from build123d import *

# Parameters (mm, degrees)
SKETCH1_R               = 1.65
SKETCH1_W               = 45
SKETCH1_H               = 23.8
BOSS_EXTRUDE1_DEPTH     = 60
FILLET1_R               = 1.5
SKETCH2_W               = 2.5
SKETCH2_H               = 4.6
CUT_EXTRUDE1_DEPTH      = 10.5
FILLET2_R               = 1
CHAMFER1_SIZE           = 1
FILLET2_OF_MIRROR2_R    = 1
CHAMFER2_SIZE           = 1
CUT_EXTRUDE2_DEPTH      = 78.903850996
CUT_EXTRUDE2_DEPTH_BACK = 78.903850996


with BuildPart() as part:
    # Sketch1 → Boss-Extrude1 (new body)
    with BuildSketch(Plane.XY):
        Polygon((-25, -11.7), (-37.5, -11.7), (-37.5, -16.3), (37.5, -16.3), (37.5, -11.7), (25, -11.7), (25, 11.7), (37.5, 11.7), (37.5, 16.3), (-37.5, 16.3), (-37.5, 11.7), (-25, 11.7), align=None)
        with Locations((-31.25, -13.85)):
            Circle(SKETCH1_R, mode=Mode.SUBTRACT)
        with Locations((31.25, -13.85)):
            Circle(SKETCH1_R, mode=Mode.SUBTRACT)
        with Locations((0, -0.4)):
            Rectangle(SKETCH1_W, SKETCH1_H, mode=Mode.SUBTRACT)
        with Locations((-31.25, 13.85)):
            Circle(SKETCH1_R, mode=Mode.SUBTRACT)
        with Locations((31.25, 13.85)):
            Circle(SKETCH1_R, mode=Mode.SUBTRACT)
    extrude(amount=BOSS_EXTRUDE1_DEPTH)

    # Fillet1
    fillet1_edges = [part.edges().sort_by_distance(p)[0] for p in [
        (22.5, 11.5, 30),
        (-22.5, 11.5, 30),
        (-22.5, -12.3, 30),
        (22.5, -12.3, 30),
        (-25, -11.7, 30),
        (-25, 11.7, 30),
        (25, 11.7, 30),
        (25, -11.7, 30),
    ]]
    fillet(fillet1_edges, radius=FILLET1_R)

    # Sketch2 → Cut-Extrude1 (cut)
    with BuildSketch(Plane(origin=(37.5, 0, 0), x_dir=(0, 0, -1), z_dir=(1, 0, 0))):
        with Locations((-13.65, -14)):
            Rectangle(SKETCH2_W, SKETCH2_H)
    cut_extrude1 = extrude(amount=-CUT_EXTRUDE1_DEPTH, mode=Mode.SUBTRACT)

    # Fillet2
    fillet2_edges = [part.edges().sort_by_distance(p)[0] for p in [
        (27, -14, 14.9),
        (27, -14, 12.4),
    ]]
    fillet(fillet2_edges, radius=FILLET2_R)

    # Chamfer1
    chamfer1_edges = [part.edges().sort_by_distance(p)[0] for p in [
        (37.5, -14, 12.4),
        (37.5, -14, 14.9),
    ]]
    chamfer(chamfer1_edges, length=CHAMFER1_SIZE)

    # Mirror2: Cut-Extrude1 across plane
    add(cut_extrude1.mirror(Plane(origin=(0, 0, 0), x_dir=(0, 0, 1), z_dir=(1, 0, 0))), mode=Mode.SUBTRACT)

    # Fillet2 of Mirror2
    fillet2_of_mirror2_edges = [part.edges().sort_by_distance(p)[0] for p in [
        (-27, -14, 14.9),
        (-27, -14, 12.4),
    ]]
    fillet(fillet2_of_mirror2_edges, radius=FILLET2_OF_MIRROR2_R)

    # Chamfer2
    chamfer2_edges = [part.edges().sort_by_distance(p)[0] for p in [
        (-37.5, -14, 12.4),
        (-37.5, -14, 14.9),
    ]]
    chamfer(chamfer2_edges, length=CHAMFER2_SIZE)

    # Sketch3 → Cut-Extrude2 (cut, two sides: drawn at the far end of the back side and taken through both)
    with BuildSketch(Plane.XZ.offset(16.3).offset(-CUT_EXTRUDE2_DEPTH_BACK)):
        with BuildLine():
            Line((-20, 50), (-20, 10))
            ThreePointArc((-20, 10), (-17.5, 7.5), (-15, 10))
            Line((-15, 10), (-15, 50))
            ThreePointArc((-15, 50), (-17.5, 52.5), (-20, 50))
        make_face()
        with BuildLine():
            ThreePointArc((20, 10), (17.5, 7.5), (15, 10))
            Line((15, 10), (15, 50))
            ThreePointArc((15, 50), (17.5, 52.5), (20, 50))
            Line((20, 50), (20, 10))
        make_face()
    extrude(amount=CUT_EXTRUDE2_DEPTH + CUT_EXTRUDE2_DEPTH_BACK, mode=Mode.SUBTRACT)


solid = part.part
Read the model definition and answer for the solid it produces. Units are mm, in the model's axes. A direction names the side the tool comes from. Round coordinates to 2 decimals unless told otherwise and drop trailing zeros. Loops run counter-clockwise (first coordinate to the right, second up) from the corner with the lowest first, then second, coordinate; pieces in that order, holes last.
Q1. Section A-A on y = 13.85 is taken. Write down the section's boundary in (x, z).
Q2. Section C-C on x = -31.25 is taken. Write down the section's boundary in (y, z).
Q3. Section B-B on x = 17.5 is taken. Write down the section's boundary in (y, z), and give its area (3 significant figures).
Q4. This flat-tipped pin is pushed along its axis until it touches: pin 1 (4 mm diameter, centred on y = -4.5, z = 44.5, fed in from -X). Where does it stop, or does it pass through?
Q5. Which of the six approach directions +Z, -Z, +X, -X, +Y, -Y give full straight-line access (tool end or side, diameter ignored) to faces 1 (the face through (-33.3, -14, 12.4)), 2 (the face through (-17.4, 13.9, 52.5)), 3 (the face through (0, 11.5, 30)), 4 (the face through (-32, -11.7, 30)), 5 (the face through (25, 0, 30))?
Q6. Section D-D on y = 8.5 is taken. Write down the section's boundary in (x, z), and give its area (3 significant figures).
Q7. Determine the mould class of faces 6 (the face through (29.94, 12.85, 29.58)), 7 (the face through (20, 14, 30)), 8 (the face through (-32.9, -13.8, 6.1)), 9 (the face through (-1, -16.3, 30)) for opening direction Y: released by +Y, released by -Y, zero draft, split by the parting line, or undercut.
Q8. Consider probe 1 along Y at (x, z) = (-31, 7); probe 2 along X at (y, z) = (-13.85, 5.5); probe 3 along X at (y, z) = (8, 29). Determine where each line is inside the solid, lowest interval first.
Output:
1. outline: (-37.5, 0) - (-32.9, 0) - (-32.9, 60) - (-37.5, 60) - close; (-29.6, 0) - (29.6, 0) - (29.6, 60) - (-29.6, 60) - close; (32.9, 0) - (37.5, 0) - (37.5, 60) - (32.9, 60) - close; hole (-20, 10) arc R2.5 ccw to (-15, 10) - (-15, 50) arc R2.5 ccw to (-20, 50) - close; hole (15, 10) arc R2.5 ccw to (20, 10) - (20, 50) arc R2.5 ccw to (15, 50) - close
2. outline: (-16.3, 0) - (-15.5, 0) - (-15.5, 12.4) - (-16.3, 12.4) - close; (-16.3, 14.9) - (-15.5, 14.9) - (-15.5, 60) - (-16.3, 60) - close; (-12.2, 0) - (-11.7, 0) - (-11.7, 12.4) - (-12.2, 12.4) - close; (-12.2, 14.9) - (-11.7, 14.9) - (-11.7, 60) - (-12.2, 60) - close; (11.7, 0) - (12.2, 0) - (12.2, 60) - (11.7, 60) - close; (15.5, 0) - (16.3, 0) - (16.3, 60) - (15.5, 60) - close
3. outline: (-16.3, 0) - (-12.3, 0) - (-12.3, 7.5) - (-16.3, 7.5) - close; (-16.3, 52.5) - (-12.3, 52.5) - (-12.3, 60) - (-16.3, 60) - close; (11.5, 0) - (16.3, 0) - (16.3, 7.5) - (11.5, 7.5) - close; (11.5, 52.5) - (16.3, 52.5) - (16.3, 60) - (11.5, 60) - close
3. area: 132 mm2
4. pin 1: stops at x = -25
5. face 1: -X, -Y
5. face 2: +Y, -Y
5. face 3: +Z, -Z
5. face 4: +Z, -Z, -X
5. face 5: +Z, -Z, +X
6. outline: (-25, 0) - (-22.5, 0) - (-22.5, 60) - (-25, 60) - close; (22.5, 0) - (25, 0) - (25, 60) - (22.5, 60) - close
6. area: 300 mm2
7. face 6: undercut
7. face 7: zero draft
7. face 8: undercut
7. face 9: released by -Y
8. probe 1: y = -16.3 to -15.48, -12.22 to -11.7, 11.7 to 12.22, 15.48 to 16.3
8. probe 2: x = -37.5 to -32.9, -29.6 to 29.6, 32.9 to 37.5
8. probe 3: x = -25 to -22.5, 22.5 to 25
